```python
from build123d import *

# Parameters (mm, degrees)
AUFSATZ_LINEAR_AUSTRAGEN1_DEPTH = 60
SCHNITT_LINEAR_AUSTRAGEN1_DEPTH = 4


with BuildPart() as part:
    # Skizze1 → Aufsatz-Linear austragen1 (new body)
    with BuildSketch(Plane.XY):
        Polygon((0, 0), (25, 0), (25, 3), (4, 3), align=None)
    extrude(amount=AUFSATZ_LINEAR_AUSTRAGEN1_DEPTH)

    # Skizze2 → Schnitt-Linear austragen1 (cut, through all)
    with BuildSketch(Plane(origin=(0, 3, 0), x_dir=(1, 0, 0), z_dir=(0, 1, 0))):
        with BuildLine():
            Line((25, -52.5), (17, -52.5))
            ThreePointArc((17, -52.5), (14.5, -50), (17, -47.5))
            Line((17, -47.5), (25, -47.5))
            Line((25, -47.5), (25, -52.5))
        make_face()
        with BuildLine():
            Line((25, -32.5), (17, -32.5))
            ThreePointArc((17, -32.5), (14.5, -30), (17, -27.5))
            Line((17, -27.5), (25, -27.5))
            Line((25, -27.5), (25, -32.5))
        make_face()
        with BuildLine():
            Line((25, -12.5), (17, -12.5))
            ThreePointArc((17, -12.5), (14.5, -10), (17, -7.5))
            Line((17, -7.5), (25, -7.5))
            Line((25, -7.5), (25, -12.5))
        make_face()
    extrude(amount=-SCHNITT_LINEAR_AUSTRAGEN1_DEPTH, mode=Mode.SUBTRACT)


solid = part.part
```
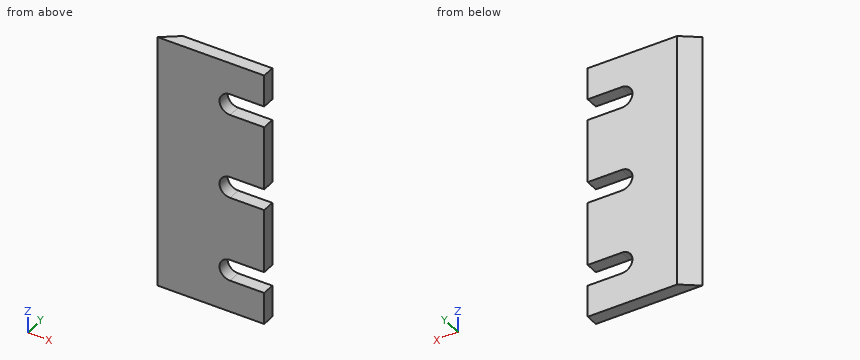
Geometry: final body of the model. Coordinates: model frame, mm. Round coordinates to 2 decimals unless told otherwise and drop trailing zeros. Loops run counter-clockwise (first coordinate to the right, second up) from the corner with the lowest first, then second, coordinate; pieces in that order, holes last.
Item 1: Section C-C, the plane z = 41.5. Output: boundary loops of the cut face in (x, y), plus the area to 3 significant figures.
Checked values:
outline: (0, 0) - (25, 0) - (25, 3) - (4, 3) - close
area: 69.0 mm2
Item 2: Section D-D, the plane x = 2. Output: boundary loops of the cut face in (y, z).
Checked values:
outline: (0, 0) - (1.5, 0) - (1.5, 60) - (0, 60) - close
Item 3: Section B-B, the plane y = 1.5. Output: boundary loops of the cut face in (x, z), plus the area to 3 significant figures.
Checked values:
outline: (2, 0) - (25, 0) - (25, 7.5) - (17, 7.5) arc R2.5 cw to (17, 12.5) - (25, 12.5) - (25, 27.5) - (17, 27.5) arc R2.5 cw to (17, 32.5) - (25, 32.5) - (25, 47.5) - (17, 47.5) arc R2.5 cw to (17, 52.5) - (25, 52.5) - (25, 60) - (2, 60) - close
area: 1,230 mm2
Item 4: Line query: L1, parallel to Z at x = 20.25, y = 2.4; L2, parallel to Z at x = 15, y = 2.75; L3, parallel to X at y = 0.9, z = 8. Output: solid intervals per line, ascending.
Checked values:
L1: z = 0 to 7.5, 12.5 to 27.5, 32.5 to 47.5, 52.5 to 60
L2: z = 0 to 8.5, 11.5 to 28.5, 31.5 to 48.5, 51.5 to 60
L3: x = 1.2 to 15.5
Item 5: Section A-A, the plane x = 17.75. Output: boundary loops of the cut face in (y, z).
Checked values:
outline: (0, 0) - (3, 0) - (3, 7.5) - (0, 7.5) - close; (0, 12.5) - (3, 12.5) - (3, 27.5) - (0, 27.5) - close; (0, 32.5) - (3, 32.5) - (3, 47.5) - (0, 47.5) - close; (0, 52.5) - (3, 52.5) - (3, 60) - (0, 60) - close
Item 6: Contact query for a flat-ended pin moving along its axis: P1, Ø1.5, axis at y = 2.5, z = 23.5, coming from the -X side. Output: stop coordinate, or through.
Checked values:
P1: stops at x = 2.33
